Autodesk Inventor part; units mm, degrees
ref_plane "YZ Plane" through (0, 0, 0) normal (1, 0, 0) x (0, 1, 0)
ref_plane "XZ Plane" through (0, 0, 0) normal (0, 1, 0) x (-1, 0, 0)
ref_plane "XY Plane" through (0, 0, 0) normal (0, 0, 1) x (1, 0, 0)
sketch "Sketch1" plane through (0, 0, 0) normal (0, 1, 0) x (-1, 0, 0)
  line L0 (0, 0) -> (107, 0)
  line L1 (107, 0) -> (107, 30)
  line L2 (107, 30) -> (42, 30)
  line L3 (0, 20) -> (0, 0)
  line L4 (42, 30) -> (42, 20)
  line L5 (42, 20) -> (0, 20)
  circle A0 centre (62, 15) radius 7.5
  circle A1 centre (92, 15) radius 4
  dimension "d6" = 15
  dimension "d7" = 8
extrude "Extrusion1" add sketch "Sketch1" along normal blind 55
sketch "Sketch2" plane through (-107, 0, 30) normal (0, 0, 1) x (1, 0, 0)
  line L0 (0, 55) -> (25, 55)
  line L1 (25, 55) -> (25, 15)
  line L2 (25, 15) -> (0, 15)
  line L3 (0, 15) -> (0, 55)
  point P0 (107, 0)
  dimension "d10" = 25
  dimension "d11" = 40
extrude "Extrusion2" cut sketch "Sketch2" against normal blind 55
sketch "Sketch3" plane through (-42, 0, 20) normal (0, 0, 1) x (1, 0, 0)
  line L0 (0, 55) -> (42, 55)
  line L1 (42, 55) -> (42, 40)
  line L2 (42, 40) -> (0, 40)
  line L3 (0, 40) -> (0, 55)
  circle A0 centre (21, 20) radius 12
  circle A1 centre (6.2237, 35.5013) radius 1.5
  circle A2 centre (36.5, 35.5) radius 1.5
  circle A3 centre (36.2237, 5.5013) radius 1.5
  circle A4 centre (6.2237, 5.5013) radius 1.5
  dimension "d14" = 42
  dimension "d15" = 15
  dimension "d16" = 24
  dimension "d22" = 3
  dimension "d23" = 3
  dimension "d24" = 3
  dimension "d25" = 3
extrude "Extrusion3" cut sketch "Sketch3" against normal blind 55
sketch "Sketch4" plane through (-42, 0, 20) normal (0, 0, 1) x (1, 0, 0)
  line L0 (42, 40) -> (0, 40)
  line L1 (0, 0) -> (0, 40)
  line L2 (0, 0) -> (42, 0)
  line L3 (42, 0) -> (42, 40)
  circle A0 centre (21, 20) radius 12
  circle A1 centre (36.2237, 5.5013) radius 1.5
  circle A2 centre (6.2237, 35.5013) radius 1.5
  circle A3 centre (36.5, 35.5) radius 1.5
  circle A4 centre (6.2237, 5.5013) radius 1.5
extrude "Extrusion4" add sketch "Sketch4" along normal blind 10
sketch "Sketch5" plane through (0, 0, 0) normal (0, 0, -1) x (-1, 0, 0)
  line L0 (42, 40) -> (0, 40)
  line L1 (0, 0) -> (0, 40)
  line L2 (0, 0) -> (107, 0)
  circle A0 centre (35.7763, 5.5013) radius 1.5
  circle A1 centre (5.5, 35.5) radius 1.5
  circle A2 centre (35.7763, 35.5013) radius 1.5
  circle A3 centre (5.7763, 5.5013) radius 1.5
  circle A4 centre (21, 20) radius 12
  line L3 (42, 40) -> (42, 0)
extrude "Extrusion5" cut sketch "Sketch5" against normal blind 20
properties part number "X_Top_MotorSide_V3" material "Birch"
Here's how the part is built. I have some questions about the finished solid (model axes, mm). A direction names the side the tool comes from. Give positions to 0.01 mm unless a question says otherwise; leave off trailing zeros. Write each loop counter-clockwise with the first axis right and the second up, starting at its lowest first coordinate (ties: lowest second). Pieces come first, ordered by that corner, then holes. Notation, with made-up numbers: M -8,79 L 3,79 A24 cw 3,111 Z; hole C -37,-29.5 d5. An arc over 180 degrees is marked long. Put each result on its own line as item: value. Start each with the question number.
Item 1: If we section it at B-B, the plane z = 21: Write out the boundary of the cut face in (x, y), then the cut area to 3 significant figures.
Item 2: If we section it at C-C, the plane x = -92: Write out the boundary of the cut face in (y, z), then the cut area to 3 significant figures.
Item 3: I need wall thicknesses on L1, parallel to X at y = 3.5, z = 18.25; L2, parallel to Y at x = -5.5, z = 22.75; L3, parallel to Z at x = -92, y = 14.5. Which ranges of each line are inside material? Lowest first, please. Write a range as from..to.
Item 4: On a 3-axis mill with a long thin cutter (end or side, diameter ignored), from which of +Z, -Z, +X, -X, +Y, -Y can I reach the whole of each face in a straight line? I mean faces 4 (the flat face through (-30, 29, 20)), 5 (the flat face through (-82, 35, 15)), 6 (the flat face through (-21, 40, 25)). Say none if no direction works.
Item 5: Thinking about a two-plate mould opening in X: for faces 1 (the cylindrical face through (-89.05, 7.4, 12.3)), 2 (the flat face through (-42, 28, 11)), 3 (the flat face through (-97, 15, 15)), which applies, +X half, -X half, draft (parallel to the pull), parting line (faces both ways), or undercut?
Item 6: Will these pins go through, and if not, where does the flat tip stop? pin 1 (1.5 mm diameter, centred on y = 22, z = 13, fed in from +X); pin 2 (10.5 mm diameter, centred on x = -92, z = 15, fed in from -Y); pin 3 (11 mm diameter, centred on x = -24, z = 26, fed in from +Y); pin 4 (20 mm diameter, centred on x = -18, y = 22, fed in from -Z).
Item 7: If we section it at A-A, the plane y = 20: Write out the boundary of the cut face in (x, z), then the cut area to 3 significant figures.
Item 8: If we section it at D-D, the plane y = 44.5: Write out the boundary of the cut face in (x, z).
Values:
1. outline: M -107,0 L -66.5,0 L -66.5,55 L -82,55 L -82,15 L -107,15 Z; M -57.5,0 L 0,0 L 0,40 L -42,40 L -42,55 L -57.5,55 Z; hole C -35.78,5.5 d3; hole C -35.78,35.5 d3; hole C -21,20 d24; hole C -5.78,5.5 d3; hole C -5.5,35.5 d3
1. area: 3,280 mm²
2. outline: M 0,0 L 15,0 L 15,11 L 0,11 Z; M 0,19 L 15,19 L 15,30 L 0,30 Z
2. area: 330 mm²
3. L1: -107..-94.33, -89.67..-68.76, -55.24..-42
3. L2: 0..4.03, 6.98..34, 37..40
3. L3: 0..11, 19..30
4. face 4: -Z, +X, +Y, -Y
4. face 5: +Z, -Z, -X, +Y
4. face 6: +Z, -Z, +X, +Y
5. face 1: undercut
5. face 2: +X half
5. face 3: draft
6. pin 1: x = -42
6. pin 2: y = 0
6. pin 3: y = 40
6. pin 4: z = 20
7. outline: M -82,0 L -42,0 L -42,20 L -33,20 L -33,30 L -82,30 Z; M -9,20 L 0,20 L 0,30 L -9,30 Z; hole C -62,15 d15
7. area: 1,200 mm²
8. outline: M -82,0 L -42,0 L -42,30 L -82,30 Z; hole C -62,15 d15
